For this review, take the finished solid that the model builds, in its own axes (mm). Face numbers are marked on the shaded views. A direction names the side the tool comes from. Round coordinates to 2 decimals unless told otherwise and drop trailing zeros. Order: outer loops, then holes, each group sorted by start corner. A loop starts at its lowest first (then second) coordinate and runs counter-clockwise, first axis right, second up. Notation, with made-up numbers: (-32.75, 4.25) -> (-5.75, 4.25) arc R15 cw to (-5.75, 30.25) -> close; hole circle Ø11 at (-18.5, 43). An arc over 180 degrees is marked (long way). Answer in a Markdown table with one row per item.
```python
from build123d import *

# Parameters (mm, degrees)
F1_DEPTH = 53.975
F3_R     = 25.4
F4_DEPTH = 76.2
F5_R     = 19.05
F6_DEPTH = 63.5
F7_R     = 12.7


with BuildPart() as f1:
    # F0 (on Top) → F1 (new body)
    with BuildSketch(Plane.XY):
        Polygon((-76.22182, -30.145772), (50.77818, -30.145772), (50.77818, 11.129228), (76.17818, 11.129228), (101.57818, 122.254228), (-76.22182, 122.254228), align=None)
    extrude(amount=F1_DEPTH)

    # F3 (on face) → F4 (join)
    with BuildSketch(Plane.XY.offset(53.975)):
        with Locations((-12.72182, 58.754228)):
            Circle(F3_R)
    extrude(amount=F4_DEPTH)

    # F5 (on face) → F6 (cut)
    with BuildSketch(Plane.XY.offset(130.175)):
        with Locations((-12.72182, 58.754228)):
            Circle(F5_R)
    extrude(amount=-F6_DEPTH, mode=Mode.SUBTRACT)

    # F7
    f7_edges = [f1.edges().sort_by_distance(p)[0] for p in [
        (-12.72182, -30.145772, 53.975),
        (50.77818, -9.508272, 53.975),
        (-76.22182, 46.054228, 53.975),
        (-38.12182, 58.754228, 53.975),
    ]]
    fillet(f7_edges, radius=F7_R)


solid = f1.part
```
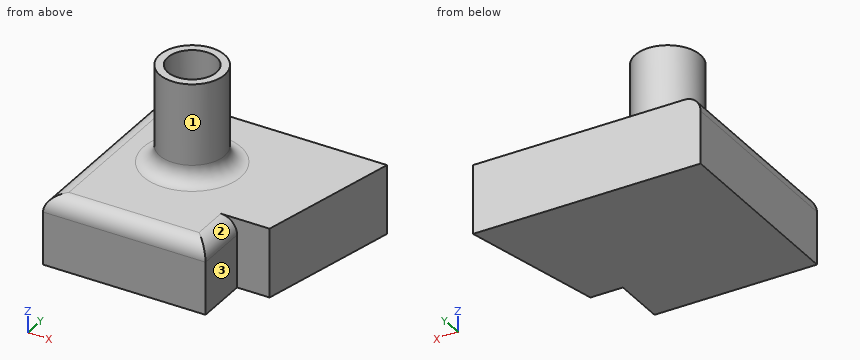
Q1. Take a section at C-C, the plane y = 17.5. Write out the cut boundary in (x, z) (3 decimals), then the cut area to 3 significant figures.
Answer key:
| item | result |
|---|---|
| outline | (-76.222, 0) -> (77.634, 0) -> (77.634, 53.975) -> (-63.522, 53.975) arc R12.7 ccw to (-76.222, 41.275) -> close |
| area | 8,270 mm^2 |
Q2. Tool access review of the marked faces 1, 2 and 3: name each direction out of +Z, -Z, +X, -X, +Y, -Y from which nothing blocks a thin tool from reaching the whole face with its end or side.
Answer key:
| item | result |
|---|---|
| face 1 | +Z |
| face 2 | +Z, +X, -Y |
| face 3 | +Z, -Z, +X, -Y |
Q3. To check wall thickness, follow probe 1 along Z at (x, y) = (25, 1) (3 decimals); probe 2 along Y at (x, z) = (71.5, 42.5); probe 3 along X at (y, z) = (-9.5, 23.5). State the ranges of each line that lie inside material, in increasing order.
Answer key:
| item | result |
|---|---|
| probe 1 | z = 0 to 53.975 |
| probe 2 | y = 11.13 to 122.25 |
| probe 3 | x = -76.22 to 50.78 |
Q4. Clearance check with flat-ended pins moving along their axes: pin 1 Ø5 at (x, y) = (40.5, 25.5) entering from -Z; pin 2 Ø1.5 at (x, y) = (-27.5, 28.5) entering from +Z; pin 3 Ø3 at (x, z) = (8, 51.5) entering from -Y; pin 4 Ø1.5 at (x, y) = (57, 105) entering from +Z (3 decimals). State where each tip first meets the part, or that it passes through.
Answer key:
| item | result |
|---|---|
| pin 1 | stops at z = 0 |
| pin 2 | stops at z = 55.08 |
| pin 3 | stops at y = -26.67 |
| pin 4 | stops at z = 53.975 |
Q5. Take a section at B-B, the plane x = 47.5. Write out the cut boundary in (y, z) (3 decimals).
Answer key:
| item | result |
|---|---|
| outline | (-30.146, 0) -> (122.254, 0) -> (122.254, 53.975) -> (11.129, 53.975) -> (11.129, 49.791) -> (-26.868, 49.791) arc R12.7 ccw to (-30.146, 41.275) -> close |
Q6. Take a section at D-D, the plane z = 70. Write out the cut boundary in (x, y).
Answer key:
| item | result |
|---|---|
| outline | circle Ø50.8 at (-12.72, 58.75); hole circle Ø38.1 at (-12.72, 58.75) |
Q7. Take a section at A-A, the plane z = 17. Write out the cut boundary in (x, y).
Answer key:
| item | result |
|---|---|
| outline | (-76.22, -30.15) -> (50.78, -30.15) -> (50.78, 11.13) -> (76.18, 11.13) -> (101.58, 122.25) -> (-76.22, 122.25) -> close |
